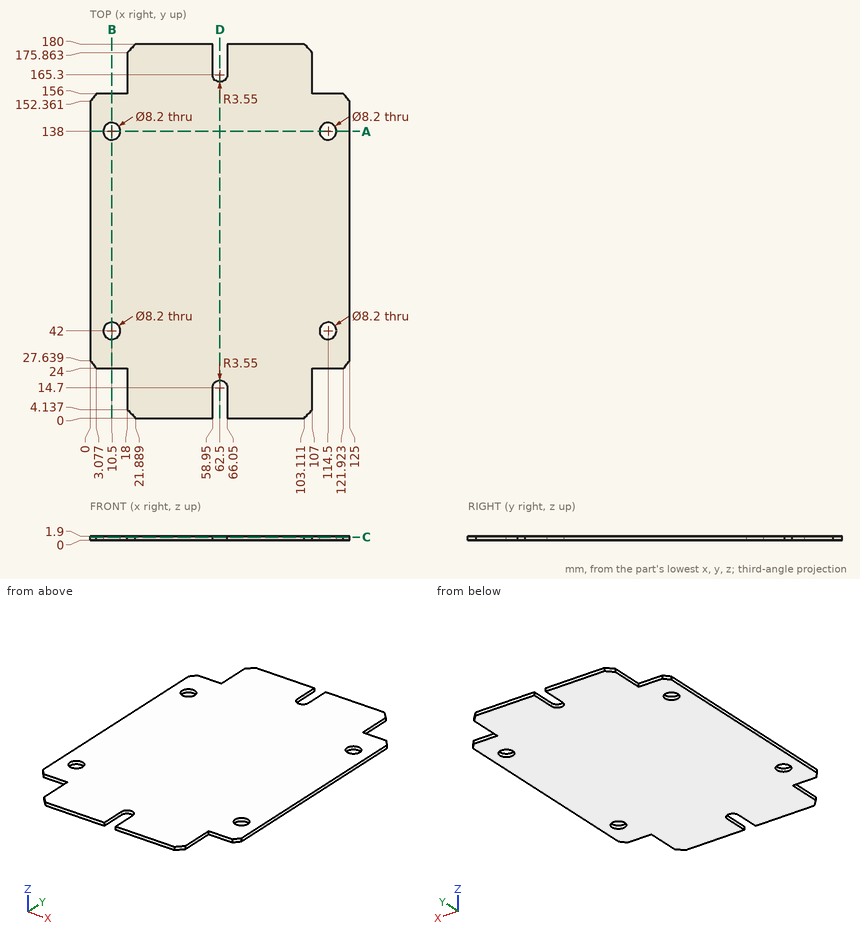
Verification items for this drawing (mm, ordinates from the low corner). Give positions to 0.01 mm unless a question says otherwise; leave off trailing zeros. Loops run counter-clockwise (first coordinate to the right, second up) from the corner with the lowest first, then second, coordinate; pieces in that order, holes last. Notation, with made-up numbers: M 15,-14.5 L 60,-14.5 A23 ccw 60,10.5 Z; hole C 46.5,78 d1. An arc over 180 degrees is marked long. Answer in a Markdown table with one row per item.
1) Thickness scan on line 1 (X direction, y = 138, z = 0.6); line 2 (Y direction, x = 114.5, z = 0.65); line 3 (X direction, y = 40.5, z = 1.15) (1 decimal). Record the ranges inside material, lowest first.
Solutions:
| item | result |
|---|---|
| line 1 | x = 0 to 6.4, 14.6 to 110.4, 118.6 to 125 |
| line 2 | y = 24 to 37.9, 46.1 to 133.9, 142.1 to 156 |
| line 3 | x = 0 to 6.7, 14.3 to 110.7, 118.3 to 125 |
2) Cross-section at D-D (x = 62.5). Enter the section's corners in (y, z).
Solutions:
| item | result |
|---|---|
| outline | M 18.25,0 L 161.75,0 L 161.75,1.9 L 18.25,1.9 Z |
3) Cross-section at C-C (z = 1.4). Count the separate pieces of the cut face and the enclosed holes in it, plus the area to 3 significant figures.
Solutions:
| item | result |
|---|---|
| separate pieces | 1 |
| enclosed holes | 4 |
| area | 20,300 mm^2 |
4) Cross-section at A-A (y = 138). Enter the section's corners in (x, z).
Solutions:
| item | result |
|---|---|
| outline | M 0,0 L 6.4,0 L 6.4,1.9 L 0,1.9 Z; M 14.6,0 L 110.4,0 L 110.4,1.9 L 14.6,1.9 Z; M 118.6,0 L 125,0 L 125,1.9 L 118.6,1.9 Z |
5) Cross-section at B-B (x = 10.5). Enter the section's corners in (y, z), plus the area to 3 significant figures.
Solutions:
| item | result |
|---|---|
| outline | M 24,0 L 37.9,0 L 37.9,1.9 L 24,1.9 Z; M 46.1,0 L 133.9,0 L 133.9,1.9 L 46.1,1.9 Z; M 142.1,0 L 156,0 L 156,1.9 L 142.1,1.9 Z |
| area | 220 mm^2 |
6) Depth check by flat-ended pin: pin 1 (1 mm diameter, centred on y = 174, z = 0.5, fed in from -X); pin 2 (0.6 mm diameter, centred on x = 112, z = 0.5, fed in from +Y); pin 3 (1 mm diameter, centred on x = 116.5, z = 0.5, fed in from -Y). Enter the tip coordinate at first touch or a pass-through.
Solutions:
| item | result |
|---|---|
| pin 1 | stops at x = 18 |
| pin 2 | stops at y = 156 |
| pin 3 | stops at y = 24 |
